Model file for the job. Use its own axes, mm. A direction names the side the tool comes from. Coordinates: 2 decimals unless noted, no trailing zeros. Write each loop counter-clockwise with the first axis right and the second up, starting at its lowest first coordinate (ties: lowest second). Pieces come first, ordered by that corner, then holes. Notation, with made-up numbers: M 25.5,50 L 32.5,50 A28 ccw 32.5,87 Z; hole C 19,-7.75 d2. An arc over 180 degrees is marked long. One line per question, with ' | ' between items. Start each with the question number.
(1) Flat gauge pins, fed straight in: pin 1 Ø0.9 at (x, z) = (0, -2) entering from -Y; pin 2 Ø1 at (y, z) = (5, -2) entering from -X; pin 3 Ø1.8 at (x, z) = (-0.5, -2) entering from +Y. Where does each tip first touch, or does it go through?
(2) Two-plate mould, pull along Y, no slides. Class faces 6 (the face through (9, -0.7, -0.3)), 7 (the face through (7.626, -4.487, -2.009)), 8 (the face through (-14.83, 5.674, -0.197)): +Y half, -Y half, draft (parallel to the pull), parting line (faces both ways), or undercut.
(3) Cut at C-C (y = -0.5). Count the separate pieces of the cut face and the enclosed holes in it, plus the area to 3 significant figures.
(4) Wall check: probe 1 along Y at (x, z) = (-5, -1.8); probe 2 along X at (y, z) = (3.5, -2.25); probe 3 along X at (y, z) = (3.25, -2.4). Give the ranges that are in metal, low to high.
(5) Cut at A-A (z = -2.4). Write the cut outline in (x, y) (3 decimals).
(6) Cut at B-B (x = -3). Write the cut outline in (y, z) (3 decimals).
(7) Cut at D-D (x = 13). Write the cut outline in (y, z) (3 decimals), plus the area to 3 significant figures.
(8) Tool access for faces 1 (the face through (0, -5.4, -2)), 2 (the face through (9.176, -0.683, -2.009)), 3 (the face through (7.691, 3.295, -3.856)), 4 (the face through (0.08, 5.27, -0.26)), 5 (the face through (0, 5.4, -2)): list every direction of +Z, -Z, +X, -X, +Y, -Y with a clear straight run to the whole face (end or side of a thin tool).
from build123d import *

# Parameters (mm, degrees)
PAD002_DEPTH            = 0.4
SKETCH005_R             = 2
POCKET002_DEPTH         = 5
PAD003_DEPTH            = 3.85
POCKET003_DEPTH         = 4.251
POCKET004_DEPTH         = 3.45
FILLET003_R             = 0.7
FILLET004_R             = 0.5
FILLET005_R             = 1.1
FILLET006_R             = 0.9
BODY001_PLACEMENT_ANGLE = 180


with BuildPart() as part:
    # Sketch004 → Pad002 (new body)
    with BuildSketch(Plane.XY):
        with BuildLine():
            Line((-13.4, 6.275), (13.4, 6.275))
            ThreePointArc((15.4, 4.275), (14.814214, 5.689214), (13.4, 6.275))
            Line((15.4, 4.275), (15.4, -4.275))
            ThreePointArc((13.4, -6.275), (14.814214, -5.689214), (15.4, -4.275))
            Line((13.4, -6.275), (-13.4, -6.275))
            ThreePointArc((-15.4, -4.275), (-14.814214, -5.689214), (-13.4, -6.275))
            Line((-15.4, -4.275), (-15.4, 4.275))
            ThreePointArc((-13.4, 6.275), (-14.814214, 5.689214), (-15.4, 4.275))
        make_face()
    extrude(amount=PAD002_DEPTH)

    # Sketch005 (on Face10 of Pad002) → Pocket002 (cut)
    with BuildSketch(Plane.XY.offset(0.4)):
        with Locations((-12.495, 0)):
            Circle(SKETCH005_R)
        with Locations((12.495, 0)):
            Circle(SKETCH005_R)
    extrude(amount=-POCKET002_DEPTH, mode=Mode.SUBTRACT)

    # Sketch006 (on Face5 of Pocket002) → Pad003 (join)
    with BuildSketch(Plane.XY.offset(0.4)):
        with BuildLine():
            Line((-5.72, 5.4), (5.72, 5.4))
            ThreePointArc((9.462119, 0.939282), (8.631248, 4.04226), (5.72, 5.4))
            Line((9.462119, 0.939282), (8.897119, -2.260718))
            ThreePointArc((5.155, -5.4), (7.59726, -4.511248), (8.897119, -2.260718))
            Line((5.155, -5.4), (-5.155, -5.4))
            ThreePointArc((-8.897119, -2.260718), (-7.59726, -4.511248), (-5.155, -5.4))
            Line((-8.897119, -2.260718), (-9.462119, 0.939282))
            ThreePointArc((-5.72, 5.4), (-8.631248, 4.04226), (-9.462119, 0.939282))
        make_face()
    extrude(amount=PAD003_DEPTH)

    # Sketch007 (on Face21 of Pad003) → Pocket003 (cut, through all)
    with BuildSketch(Plane.XY.offset(4.25)):
        with BuildLine():
            Line((-5.72, 4.2), (5.72, 4.2))
            ThreePointArc((8.280397, 1.14793), (7.711906, 3.27102), (5.72, 4.2))
            Line((8.280397, 1.14793), (7.715397, -2.05207))
            ThreePointArc((5.155, -4.2), (6.82602, -3.591906), (7.715397, -2.05207))
            Line((5.155, -4.2), (-5.155, -4.2))
            ThreePointArc((-7.715397, -2.05207), (-6.82602, -3.591906), (-5.155, -4.2))
            Line((-7.715397, -2.05207), (-8.280397, 1.14793))
            ThreePointArc((-5.72, 4.2), (-7.711906, 3.27102), (-8.280397, 1.14793))
        make_face()
    extrude(amount=-POCKET003_DEPTH, mode=Mode.SUBTRACT)

    # Sketch008 (on Face4 of Pocket003) → Pocket004 (cut)
    with BuildSketch(Plane(origin=(0, 0, 0), x_dir=(1, 0, 0), z_dir=(0, 0, -1))):
        with BuildLine():
            Line((-5.155, 5), (5.155, 5))
            ThreePointArc((8.503211, 2.191169), (7.34018, 4.204801), (5.155, 5))
            Line((8.503211, 2.191169), (9.068211, -1.008831))
            ThreePointArc((5.72, -5), (8.324801, -3.78518), (9.068211, -1.008831))
            Line((5.72, -5), (-5.72, -5))
            ThreePointArc((-9.068211, -1.008831), (-8.324801, -3.78518), (-5.72, -5))
            Line((-9.068211, -1.008831), (-8.503211, 2.191169))
            ThreePointArc((-5.155, 5), (-7.34018, 4.204801), (-8.503211, 2.191169))
        make_face()
    extrude(amount=-POCKET004_DEPTH, mode=Mode.SUBTRACT)

    # Fillet003
    fillet003_edges = [part.edges().sort_by_distance(p)[0] for p in [
        (8.324801, 3.78518, 3.45),
    ]]
    fillet(fillet003_edges, radius=FILLET003_R)

    # Fillet004
    fillet004_edges = [part.edges().sort_by_distance(p)[0] for p in [
        (8.631248, 4.04226, 0.4),
    ]]
    fillet(fillet004_edges, radius=FILLET004_R)

    # Fillet005
    fillet005_edges = [part.edges().sort_by_distance(p)[0] for p in [
        (8.631248, 4.04226, 4.25),
    ]]
    fillet(fillet005_edges, radius=FILLET005_R)

    # Fillet006
    fillet006_edges = [part.edges().sort_by_distance(p)[0] for p in [
        (0, 5, 0),
    ]]
    fillet(fillet006_edges, radius=FILLET006_R)


with BuildPart() as part_1:
    # Body001 placement: moved
    add(part.part.rotate(Axis((0, 0, 0), (0, 1, 0)), BODY001_PLACEMENT_ANGLE))


solid = part_1.part
Filled in:
1) pin 1: y = -5.4 | pin 2: x = -8.18 | pin 3: y = 5.4
2) face 6: undercut | face 7: -Y half | face 8: +Y half
3) separate pieces: 4 | enclosed holes: 0 | area: 6.05 mm²
4) probe 1: -5.4 to -5, 5 to 5.4 | probe 2: -9.01 to -8.54, 8.54 to 9.01 | probe 3: -9.14 to -8.69, 8.69 to 9.14
5) outline: M -9.462,0.939 L -8.897,-2.261 A3.8 ccw -5.155,-5.4 L 5.155,-5.4 A3.8 ccw 8.897,-2.261 L 9.462,0.939 A3.8 ccw 5.72,5.4 L -5.72,5.4 A3.8 ccw Z; hole M -9.068,1.009 L -8.503,-2.191 A3.4 ccw -5.155,-5 L 5.155,-5 A3.4 ccw 8.503,-2.191 L 9.068,1.009 A3.4 ccw 5.72,5 L -5.72,5 A3.4 ccw Z
6) outline: M -6.275,-0.4 L -5.9,-0.4 A0.5 cw -5.4,-0.9 L -5.4,-3.15 A1.1 ccw -4.3,-4.25 L -4.2,-4.25 L -4.2,-3.45 L -4.3,-3.45 A0.7 cw -5,-2.75 L -5,-0.9 A0.9 ccw -5.9,0 L -6.275,0 Z; M 4.2,-4.25 L 4.3,-4.25 A1.1 ccw 5.4,-3.15 L 5.4,-0.9 A0.5 cw 5.9,-0.4 L 6.275,-0.4 L 6.275,0 L 5.9,0 A0.9 ccw 5,-0.9 L 5,-2.75 A0.7 cw 4.3,-3.45 L 4.2,-3.45 Z
7) outline: M -6.275,-0.4 L -1.935,-0.4 L -1.935,0 L -6.275,0 Z; M 1.935,-0.4 L 6.275,-0.4 L 6.275,0 L 1.935,0 Z | area: 3.47 mm²
8) face 1: -Z, +X, -X, -Y | face 2: -Z, +X, -Y | face 3: +Z, -Z | face 4: +Z | face 5: -Z, +X, -X, +Y
